from build123d import *

# Parameters (mm, degrees)
SKETCH1_W           = 37
SKETCH1_H           = 80
BOSS_EXTRUDE1_DEPTH = 2
SKETCH2_W           = 0.9
SKETCH2_H           = 1.5
BOSS_EXTRUDE2_DEPTH = 80
SKETCH3_W           = 29.726914408
SKETCH3_H           = 4
CUT_EXTRUDE1_DEPTH  = 2


with BuildPart() as part:
    # Sketch1 → Boss-Extrude1 (new body)
    with BuildSketch(Plane.XY):
        with Locations((18.5, 40)):
            Rectangle(SKETCH1_W, SKETCH1_H)
    extrude(amount=BOSS_EXTRUDE1_DEPTH)

    # Sketch2 → Boss-Extrude2 (add)
    with BuildSketch(Plane(origin=(0, 80, 0), x_dir=(1, 0, 0), z_dir=(0, 1, 0))):
        with Locations((37.45, -1)):
            Rectangle(SKETCH2_W, SKETCH2_H)
        with Locations((-0.45, -1)):
            Rectangle(SKETCH2_W, SKETCH2_H)
    extrude(amount=-BOSS_EXTRUDE2_DEPTH)

    # Sketch3 → Cut-Extrude1 (cut)
    with BuildSketch(Plane.XY.offset(2)):
        with Locations((18.5, 2)):
            Rectangle(SKETCH3_W, SKETCH3_H)
    extrude(amount=-CUT_EXTRUDE1_DEPTH, mode=Mode.SUBTRACT)


solid = part.part
Input: part model. Units: mm. Frame: model coordinates. A direction names the side the tool comes from. Give positions to 0.01 mm unless a question says otherwise; leave off trailing zeros. Write each loop counter-clockwise with the first axis right and the second up, starting at its lowest first coordinate (ties: lowest second). Pieces come first, ordered by that corner, then holes.
Q1. Set-up query: faces 4 (the face through (3.637, 2, 1)), 5 (the face through (1, 0, 1)). Return all of +Z, -Z, +X, -X, +Y, -Y with unobstructed straight access to the full face (end or side cutting, diameter ignored); none if empty.
Q2. Pull-direction query (X, two-part tool) for faces 1 (the face through (37.9, 41, 1)), 2 (the face through (18, 41, 0)), 3 (the face through (18, 4, 1)); classes: pulls with the +X half, pulls with the -X half, needs draft (parallel to the pull), parting line crosses it, or undercut.
Q3. Material intervals for probe 1 along Y at (x, z) = (15, 1.75); probe 2 along X at (y, z) = (10, 0.2), sorted ascending.
Q4. First-contact query: P1, Ø0.7, axis at x = 37.5, y = 54, coming from the +Z side; P2, Ø0.7, axis at x = 37.5, y = 47.5, coming from the -Z side. Flat tips, straight axial feed; report the tip coordinate or a pass-through.
Q5. Section B-B, the plane x = 9. Output: boundary loops of the cut face in (y, z).
Q6. Section A-A, the plane z = 0.65. Output: boundary loops of the cut face in (x, y).
Filled in:
1. face 4: +Z, -Z, -Y
1. face 5: +Z, -Z, +X, -X, -Y
2. face 1: pulls with the +X half
2. face 2: needs draft
2. face 3: undercut
3. probe 1: y = 4 to 80
3. probe 2: x = 0 to 37
4. P1: stops at z = 1.75
4. P2: stops at z = 0.25
5. outline: (4, 0) - (80, 0) - (80, 2) - (4, 2) - close
6. outline: (-0.9, 0) - (3.64, 0) - (3.64, 4) - (33.36, 4) - (33.36, 0) - (37.9, 0) - (37.9, 80) - (-0.9, 80) - close
